Autodesk Inventor part; units mm, degrees
sketch "Sketch1" plane through (0, 0, 0) normal (1, 0, 0) x (0, 1, 0)
  circle A0 centre (30.5, -5.5) radius 3.5
  line L0 (11, 15) -> (5, 15)
  line L1 (5, -15) -> (11, -15)
  line L2 (0, -21) -> (5, -21)
  line L3 (5, -21) -> (5, -15)
  line L4 (0, 21) -> (5, 21)
  line L5 (5, 21) -> (5, 15)
  line L6 (-7.7302, 0) -> (46.3815, 0)
  line L7 (0, 29.4) -> (0, -29.4)
  line L8 (0, 21) -> (0, -21)
  line L9 (11, -15) -> (23.6512, -15)
  line L10 (11, 15) -> (23.6512, 15)
  arc A1 (23.6512, -15) -> (23.6512, 15) centre (23.6512, 0) ccw
  circle A2 centre (11, 0) radius 5
  point P0 (2.5, -21)
  dimension "d7" = 7
  dimension "d45" = 21
  dimension "d64" = 5
  dimension "d65" = 21
  dimension "d66" = 5
  dimension "d67" = 15
  dimension "d69" = 5.5
  dimension "d73" = 0
  dimension "d74" = 30.5
  dimension "d75" = 10
  dimension "d76" = 0
  dimension "d77" = 11
  dimension "d78" = 15
  dimension "d79" = 15
  dimension "d80" = 23.6512
extrude "Extrusion1" add sketch "Sketch1" along normal blind 10 contours L10 A1 L6 A2 L7 L4 L5 L0 | A1 L9 L1 L3 L2 L7 L6 A2
sketch "Sketch4" plane through (10, 0, 0) normal (1, 0, 0) x (0, 0, -1)
  circle A0 centre (0, 11) radius 9.5
  circle A1 centre (5.5, 30.5) radius 5
  line L0 (-29.4, 0) -> (29.4, 0)
  line L1 (0, -7.7302) -> (0, 46.3815)
  point P0 (0, 0)
  dimension "d56" = 19
  dimension "d57" = 10
  dimension "d58" = 11
  dimension "d59" = 0
  dimension "d60" = 30.5
  dimension "d61" = 5.5
extrude "Extrusion2" cut sketch "Sketch4" along normal blind 5 from surface at -10
sketch "Sketch6" plane through (0, 5, -15) normal (0, 1, 0) x (1, 0, 0)
  circle A0 centre (5, 3) radius 1.5
  line L0 (12, -15) -> (-2, -15)
  circle A1 centre (5, -33) radius 1.5
  line L1 (0, -30) -> (0, -36)
  line L2 (0, 6) -> (0, 0)
  point P0 (0, -15)
  point P1 (0, -33)
  point P2 (0, 3)
  dimension "d81" = 3
  dimension "d82" = 18
  dimension "d83" = 3
  dimension "d84" = 18
  dimension "d85" = 5
  dimension "d86" = 5
extrude "Extrusion3" cut sketch "Sketch6" against normal blind 5
Build history of the part. All positions in model axes, mm. A direction names the side the tool comes from. Give positions to 0.01 mm unless a question says otherwise; leave off trailing zeros. Order: outer loops, then holes, each group sorted by start corner. A loop starts at its lowest first (then second) coordinate and runs counter-clockwise, first axis right, second up. Notation, with made-up numbers: M 45,-16 L 98,-16 A18 cw 98,0 Z; hole C 33,30 d4. An arc over 180 degrees is marked long. Put each result on its own line as item: value.
Item 1: 3-axis set-ups, long thin cutter, end or side, ignore diameter. For faces 1 (the cylindrical face through (2.46, 2.99, -5.11)), 2 (the cylindrical face through (7.46, 15.77, -1.5)), 3 (the flat face through (3.8, 5, 19.4)), 4 (the flat face through (0, 23, 0)), 5 (the flat face through (5, 14, -15)): which of +Z, -Z, +X, -X, +Y, -Y reach the whole face in a straight line?
From the geometry:
face 1: -X
face 2: +X, -X
face 3: +Z, +X, -X, +Y
face 4: +Z, -Z, -X, +Y, -Y
face 5: -Z, +X, -X, +Y
Item 2: Probe line 1 (Z direction, x = 5, y = 1.1); line 2 (Y direction, x = 6.95, z = 0); line 3 (Z direction, x = 4, y = 11). List the from-to ranges inside material, lowest first. Write a range as [from, to].
From the geometry:
line 1: z = [-21, -19.5], [-16.5, 16.5], [19.5, 21]
line 2: y = [0, 6], [16, 38.65]
line 3: z = [-15, -9.5], [9.5, 15]
Item 3: Flat gauge pins, fed straight in: pin 1 Ø4 at (y, z) = (27, 11.5) entering from -X; pin 2 Ø8 at (y, z) = (30.5, -5.5) entering from -X; pin 3 Ø1.5 at (x, y) = (1.5, 30.5) entering from -Z; pin 4 Ø1.8 at (x, z) = (3.5, -16.5) entering from +Y. Where does each tip first touch, or does it go through?
From the geometry:
pin 1: stops at x = 0
pin 2: stops at x = 5
pin 3: stops at z = -13.7
pin 4: stops at y = 5
Item 4: Slice it at D-D, the plane z = 0. Write the cut outline in (x, y).
From the geometry:
outline: M 0,0 L 10,0 L 10,6 L 5,6 L 5,1.5 L 0,1.5 Z; M 0,20.5 L 5,20.5 L 5,16 L 10,16 L 10,38.65 L 0,38.65 Z
Item 5: Slice it at A-A, the plane z = 18. Write the cut outline in (x, y).
From the geometry:
outline: M 0,0 L 3.5,0 L 3.5,5 L 0,5 Z; M 6.5,0 L 10,0 L 10,5 L 6.5,5 Z
Item 6: Slice it at C-C, the plane y = 9. Write the cut outline in (x, z), plus the area to 3 significant figures.
From the geometry:
outline: M 0,-15 L 10,-15 L 10,-4.58 L 5,-4.58 L 5,-9.29 L 0,-9.29 Z; M 0,9.29 L 5,9.29 L 5,4.58 L 10,4.58 L 10,15 L 0,15 Z
area: 161 mm2
Item 7: Two-plate mould, pull along Z, no slides. Class faces 6 (the flat face through (5, 2, -21)), 7 (the flat face through (5, 2, 21)), 8 (the flat face through (5, 29, -2)): +Z half, -Z half, draft (parallel to the pull), parting line (faces both ways), or undercut.
From the geometry:
face 6: -Z half
face 7: +Z half
face 8: undercut
Item 8: Slice it at B-B, the plane x = 1.25. Write the cut outline in (y, z), plus the area to 3 significant figures.
From the geometry:
outline: M 0,-21 L 5,-21 L 5,-15 L 23.65,-15 A15 ccw 23.65,15 L 5,15 L 5,21 L 0,21 Z; hole C 11,0 d19; hole C 30.5,-5.5 d10
area: 761 mm2
